Design review of the part shown in the three views and the two pictorial views. Dimensions are in mm from the part's minimum x, y and z. A direction names the side the tool comes from. Coordinates: 2 decimals unless noted, no trailing zeros. Order: outer loops, then holes, each group sorted by start corner. A loop starts at its lowest first (then second) coordinate and runs counter-clockwise, first axis right, second up. Notation, with made-up numbers: (-22, 13) - (-8, 13) arc R17 cw to (-8, 25) - close; hole circle Ø10 at (33.5, -36.75). An arc over 180 degrees is marked (long way). One line per item, written item: value. Start each with the question number.
(1) Mouldability with a two-part tool opening along Y and no side actions: class the marked faces 5, 6, 7 and 8 as released by +Y, released by -Y, zero draft, split by the parting line, or undercut.
(2) Consider section C-C on z = 8. Write out the cut boundary in (x, y) (1 decimal), then the cut area to 3 significant figures.
(3) To check wall thickness, follow line 1 along Y through (x, z) = (11, 3) (1 decimal); line 2 along Y through (x, z) = (25, 12.5); line 3 along Z through (x, y) = (7, 22.5). State the ranges of each line that lie inside material, in increasing order.
(4) Consider section A-A on y = 53.5. Write out the cut boundary in (x, z).
(5) Clearance check with flat-ended pins moving along their axes: pin 1 (10 mm diameter, centred on y = 56, z = 12.5, fed in from -X); pin 2 (6 mm diameter, centred on x = 38, y = 84, fed in from +Z) (1 decimal); pin 3 (11.5 mm diameter, centred on x = 12.68, y = 11.96, fed in from -Z); pin 4 (10.5 mm diameter, centred on x = 13.5, y = 87.5, fed in from +Z). State where each tip first meets the part, or that it passes through.
(6) Consider section B-B on x = 37. Write out the cut boundary in (y, z).
(7) For the marked faces 1, 2, 3 and 4, list the 3-axis set-ups (+Z, -Z, +X, -X, +Y, -Y) from which the entire face can be reached by the end or side of a thin tool; tool diameter is ignored.
(8) Consider section D-D on z = 29. Write out the cut boundary in (x, y), then the cut area to 3 significant figures.
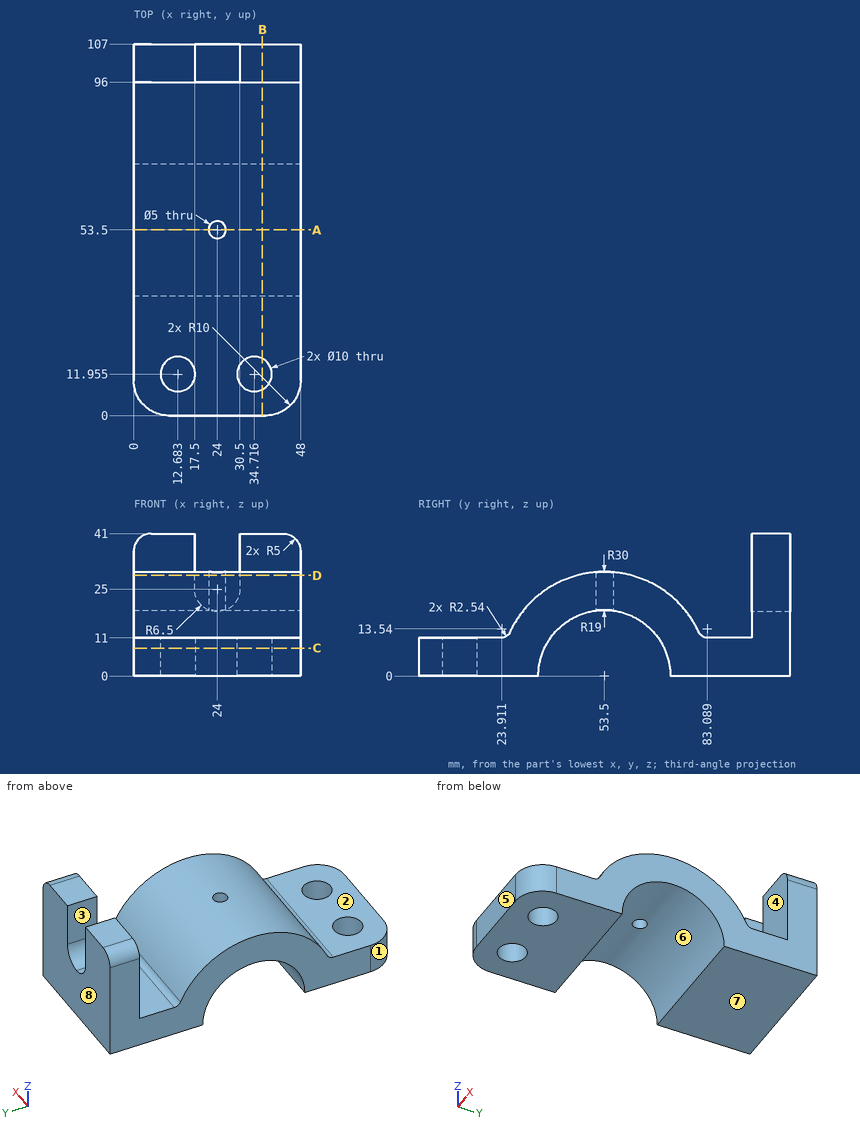
Geometry check:
1. face 5: released by -Y
1. face 6: undercut
1. face 7: zero draft
1. face 8: released by +Y
2. outline: (0, 10) arc R10 ccw to (10, 0) - (38, 0) arc R10 ccw to (48, 10) - (48, 36.3) - (0, 36.3) - close; (0, 70.7) - (48, 70.7) - (48, 107) - (0, 107) - close; hole circle Ø10 at (12.7, 12); hole circle Ø10 at (34.7, 12)
2. area: 3,280 mm^2
3. line 1: y = 0 to 7.2, 16.7 to 34.7, 72.3 to 107
3. line 2: y = 26.23 to 39.19, 67.81 to 80.77, 96 to 107
3. line 3: z = 0 to 11
4. outline: (0, 19) - (21.5, 19) - (21.5, 30) - (0, 30) - close; (26.5, 19) - (48, 19) - (48, 30) - (26.5, 30) - close
5. pin 1: passes through
5. pin 2: stops at z = 12.1
5. pin 3: stops at z = 0
5. pin 4: stops at z = 11.14
6. outline: (0, 0) - (7.51, 0) - (7.51, 11) - (0, 11) - close; (16.4, 0) - (34.5, 0) arc R19 cw to (72.5, 0) - (107, 0) - (107, 41) - (96, 41) - (96, 11) - (83.09, 11) arc R2.54 cw to (80.78, 12.48) arc R30 ccw to (26.22, 12.48) arc R2.54 cw to (23.91, 11) - (16.4, 11) - close
7. face 1: +Z, -Z, -X, -Y
7. face 2: +Z, +X, -X, -Y
7. face 3: +Z, +Y
7. face 4: +Z, +X, -X
8. outline: (0, 45.82) - (48, 45.82) - (48, 61.18) - (0, 61.18) - close; (0, 96) - (17.5, 96) - (17.5, 107) - (0, 107) - close; (30.5, 96) - (48, 96) - (48, 107) - (30.5, 107) - close; hole circle Ø5 at (24, 53.5)
8. area: 1,100 mm^2
